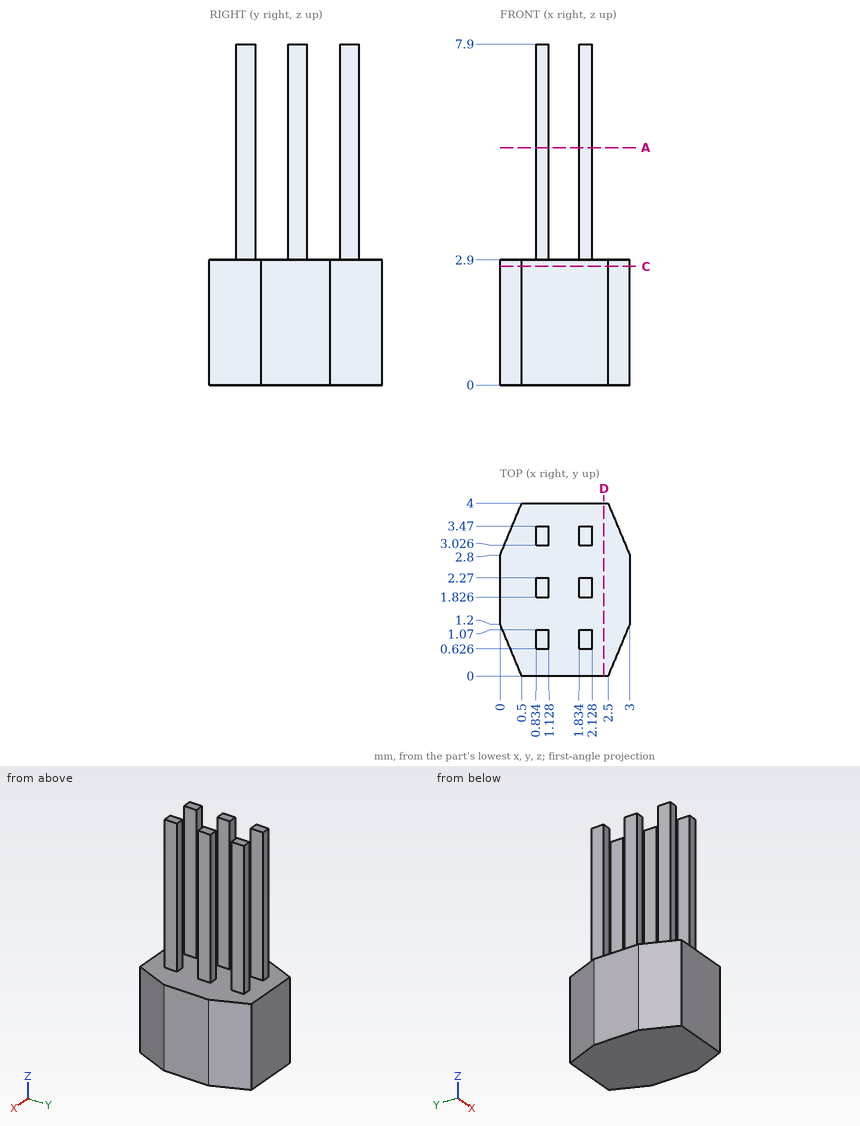
Could you check a few things on this drawing? It's one solid part, dimensions in mm from its lowest x, y, z. Coordinates: 2 decimals unless noted, no trailing zeros. Order: outer loops, then holes, each group sorted by start corner. A loop starts at its lowest first (then second) coordinate and runs counter-clockwise, first axis right, second up.
1) Imagine slicing it at D-D on x = 2.4. List the corners of the cut face in (y, z) for me.
2) Imagine slicing it at C-C on z = 2.75. List the corners of the cut face in (x, y) for me, and give its area (3 significant figures).
3) Will these pins go through, and if not, where does the flat tip stop? pin 1 (1.5 mm diameter, centred on x = 1.5, z = 4, fed in from +Y); pin 2 (0.5 mm diameter, centred on y = 0.5, z = 4.5, fed in from +X).
4) I need wall thicknesses on line 1 (Y direction, x = 2, z = 5.5) (1 decimal); line 2 (X direction, y = 0.9, z = 6.5) (1 decimal); line 3 (Z direction, x = 1.8, y = 3.25). Which ranges of each line are inside material? Lowest first, please.
5) Imagine slicing it at A-A on z = 5.5. State how many separate pieces and enclosed holes the cut face has.
Response values:
1. outline: (0, 0) - (4, 0) - (4, 2.9) - (0, 2.9) - close
2. outline: (0, 1.2) - (0.5, 0) - (2.5, 0) - (3, 1.2) - (3, 2.8) - (2.5, 4) - (0.5, 4) - (0, 2.8) - close
2. area: 10.8 mm2
3. pin 1: stops at y = 3.47
3. pin 2: stops at x = 2.13
4. line 1: y = 0.6 to 1.1, 1.8 to 2.3, 3 to 3.5
4. line 2: x = 0.8 to 1.1, 1.8 to 2.1
4. line 3: z = 0 to 2.9
5. separate pieces: 6
5. enclosed holes: 0
